from build123d import *

# Parameters (mm, degrees)
F1_DEPTH = 53.2
F2_R     = 9.7217056973
F3_DEPTH = 106.8
F4_DEPTH = 33.4


# Not quite as in the source:
# - ends of sketch curves that miss each other by under 0.0002 mm in the source are joined


with BuildPart() as f1:
    # F0 (on Top) → F1 (new body)
    with BuildSketch(Plane.XY):
        with BuildLine():
            Line((-7.9474923426, 50.9009919427), (-113.0345375872, 34.4224307572))
            ThreePointArc((-113.0345375872, 34.4224307572), (-140.0579018259, -1.5509775623), (-109.9911685167, -35.0224560031))
            Line((-109.9911685167, -35.0224560031), (-7.9210999462, -50.905094516))
            ThreePointArc((-7.9210999462, -50.905094516), (51.5176891338, 0.0133546718), (-7.9474923426, 50.9009919427))
        make_face()
        with BuildLine():
            ThreePointArc((-4.8825833147, 31.1371999002), (31.5176854276, 0.01851299), (-4.8460009605, -31.1429143167))
            Line((-4.8460009605, -31.1429143167), (-106.957762942, -15.2537880902))
            ThreePointArc((-106.957762942, -15.2537880902), (-120.0581940893, -1.0187143376), (-108.9482164871, 14.8188049967))
            Line((-108.9482164871, 14.8188049967), (-4.8825833147, 31.1371999002))
        make_face(mode=Mode.SUBTRACT)
    extrude(amount=-F1_DEPTH)

    # F2 (on face) → F3 (join)
    with BuildSketch(Plane(origin=(-7.9210999462, -50.905094516, 0), x_dir=(0.98810901, -0.1537549493, 0), z_dir=(-0.1537549493, -0.98810901, 0))):
        with Locations((-51.6491943406, -26.6)):
            Circle(F2_R)
    extrude(amount=-F3_DEPTH)

    # F4 (add): a face of the model
    f4_faces = [f1.faces().sort_by_distance(p)[0] for p in [
        (-42.5351056478, 62.5662670045, -26.6),
    ]]
    extrude(f4_faces, amount=-F4_DEPTH)


solid = f1.part
Input: part model. Units: mm. Frame: model coordinates. A direction names the side the tool comes from. Coordinates: 2 decimals unless noted, no trailing zeros. Loops run counter-clockwise (first coordinate to the right, second up) from the corner with the lowest first, then second, coordinate; pieces in that order, holes last. Notation, with made-up numbers: (7, -12) - (39, -12) arc R22 ccw to (39, -4) - close; hole circle Ø6 at (68.25, -4). An arc over 180 degrees is marked (long way). Answer in a Markdown table with one row per item. Add a question column.
Item 1: Section query B-B on z = -12. Return the cut outline in (x, y).
Item 2: Mould query, pull axis X, two halves, no side actions, for faces 1 (the cylindrical face through (-43.128, 0.352, -30.323)), 2 (the cylindrical face through (-140.08, -0.87, -26.23)), 3 (the flat face through (-67, -22, -53.2)). Classes: released by +X, released by -X, zero draft, split by the parting line, or undercut.
Item 3: Line query: line 1 along X through (y, z) = (0, -12); line 2 along Y through (x, z) = (0, -36); line 3 along X through (y, z) = (0, -27.5). Output: solid intervals per line, ascending. Write a range as [from, to].
Item 4: Contact query for flat-ended pins moving along their axis: P1, Ø1, axis at y = -27.5, z = -17.5, coming from the -X side; P2, Ø1, axis at y = 8.5, z = -33, coming from the -X side; P3, Ø1.5, axis at y = -3.5, z = -34.5, coming from the -X side. Output: stop coordinate, or through.
Item 5: Section query D-D on x = -79. Return the cut outline in (y, z).
Item 6: Section query A-A on x = 0. Return the cut outline in (y, z).
Item 7: Section query C-C on y = -4.5. State how many separate pieces and enclosed holes the cut face has, then the cut area to 3 significant figures.
Item 8: Access query for faces 4 (the cylindrical face through (-120.036, -1.311, -26.228)), 5 (the flat face through (-67, -22, 0)). Directions: +Z, -Z, +X, -X, +Y, -Y. A direction counts if a zero-diameter tool reaches every point of the face in a straight line with its end or side. Return the directions, or none.
Recorded:
| question | item | result |
|---|---|---|
| 1 | outline | (-113.03, 34.42) arc R35.42 ccw to (-109.99, -35.02) - (-7.92, -50.91) arc R51.52 ccw (long way) to (-7.95, 50.9) - close; hole (-108.95, 14.82) arc R15.42 ccw to (-106.96, -15.25) - (-4.85, -31.14) arc R31.52 ccw (long way) to (-4.88, 31.14) - close |
| 2 | face 1 | undercut |
| 2 | face 2 | released by -X |
| 2 | face 3 | zero draft |
| 3 | line 1 | [-140.09, -120.09], [31.52, 51.52] |
| 3 | line 2 | [-51.52, -31.52], [31.52, 51.52] |
| 3 | line 3 | [-140.09, -120.09], [-62.07, -42.47], [31.52, 51.52] |
| 4 | P1 | x = -127.6 |
| 4 | P2 | x = -139.18 |
| 4 | P3 | x = -139.98 |
| 5 | outline | (-39.84, -53.2) - (-19.6, -53.2) - (-19.6, 0) - (-39.84, 0) - close; (19.51, -53.2) - (39.76, -53.2) - (39.76, 0) - (19.51, 0) - close |
| 6 | outline | (-51.52, -53.2) - (-31.52, -53.2) - (-31.52, 0) - (-51.52, 0) - close; (31.52, -53.2) - (51.52, -53.2) - (51.52, 0) - (31.52, 0) - close |
| 7 | separate pieces | 3 |
| 7 | enclosed holes | 0 |
| 7 | area | 2,460 mm^2 |
| 8 | face 4 | +Z, -Z |
| 8 | face 5 | +Z, +X, -X, +Y, -Y |
